Geometry check sheet. Reference: the model listing, model coordinates, mm. A direction names the side the tool comes from. Round coordinates to 2 decimals unless told otherwise and drop trailing zeros. Write each loop counter-clockwise with the first axis right and the second up, starting at its lowest first coordinate (ties: lowest second). Pieces come first, ordered by that corner, then holes. Notation, with made-up numbers: M -17,61 L 38,61 A30 cw 38,92 Z; hole C -8,-28 d11. An arc over 180 degrees is marked long. One line per item, written item: value. Start each with the question number.
1. Section check A-A (y = -69.5). Record the boundary of the cut face in (x, z).
2. Scan lines: probe 1 along X at (y, z) = (-54.5, 4.5); probe 2 along Y at (x, z) = (100, 5.5); probe 3 along Y at (x, z) = (101.6, 7.75). Record each from-to range of solid material in increasing order. Write a range as [from, to].
3. Access from +Z, -Z, +X, -X, +Y, -Y to the whole of each face (thin tool, end or side, straight path). Record for faces 4 (the flat face through (230, 107.95, 6)), 5 (the flat face through (2, 215.9, 6)), 6 (the flat face through (-227, 107.95, 6)), 7 (the flat face through (-95.43, -12.88, 6.26)).
4. Section check B-B (x = 195). Record the boundary of the cut face in (y, z), and give its area (3 significant figures).
5. Depth check by flat-ended pin: P1, Ø6, axis at x = -239.61, y = 101.6, coming from the -Z side; P2, Ø6, axis at x = 317.5, y = 33.87, coming from the +Z side; P3, Ø4, axis at x = -114.3, y = -53.77, coming from the +Z side; P4, Ø4, axis at x = 191, z = 7.5, coming from the +Y side. Enter the tip coordinate at first touch or a pass-through.
6. Section check C-C (z = 8.75). Count the separate pieces of the cut face and the enclosed holes in it, and give its area (3 significant figures).
7. Release check for a two-part mould opening along X. For faces 1 (the flat face through (-323.85, 2, 6)), 2 (the flat face through (107.95, -66, 6)), 3 (the flat face through (214, -107.95, 6)) record: pulls with the +X half, pulls with the -X half, needs draft (parallel to the pull), parting line crosses it, or undercut.
from build123d import *

# Parameters (mm, degrees)
F0_R           = 27.94
F1_DEPTH       = 12.7
F3_D           = 4.7625
F3_CSINK_D     = 7.9375
F3_CSINK_ANGLE = 85
F4_SIZE        = 1.5875


with BuildPart() as f1:
    # F0 (on Top) → F1 (new body)
    with BuildSketch(Plane.XY):
        Polygon((-82.55, 0), (82.55, 0), (107.95, -25.4), (107.95, -107.95), (323.85, -107.95), (323.85, 107.95), (133.35, 107.95), (107.95, 133.35), (107.95, 215.9), (-107.95, 215.9), (-107.95, 133.35), (-133.35, 107.95), (-323.85, 107.95), (-323.85, -107.95), (-107.95, -107.95), (-107.95, -25.4), align=None)
        with Locations((0, 107.95)):
            Circle(F0_R, mode=Mode.SUBTRACT)
    extrude(amount=F1_DEPTH)

    # F3 (through all)
    with Locations(Plane.XY.offset(12.7)):
        with Locations((-239.609983, 101.6), (-161.719967, 101.6), (-116.159872, 116.159872), (-101.6, 161.719967), (-101.6, 209.55), (-33.866667, 209.55), (33.866667, 209.55), (101.6, 209.55), (101.6, 161.719967), (116.159872, 116.159872), (161.719967, 101.6), (239.609983, 101.6), (317.5, 33.866667), (317.5, 101.6), (317.5, -33.866667), (317.5, -101.6), (249.766667, -101.6), (182.033333, -101.6), (114.3, -53.769967), (114.3, -101.6), (99.740128, -8.209872), (54.180033, 6.35), (0, 6.35), (-54.180033, 6.35), (-99.740128, -8.209872), (-114.3, -53.769967), (-114.3, -101.6), (-182.033333, -101.6), (-249.766667, -101.6), (-317.5, -101.6), (-317.5, -33.866667), (-317.5, 33.866667), (-317.5, 101.6)):
            CounterSinkHole(F3_D / 2, F3_CSINK_D / 2, counter_sink_angle=F3_CSINK_ANGLE)

    # F4
    f4_edges = [f1.edges().sort_by_distance(p)[0] for p in [
        (-27.94, 107.95, 12.7),
    ]]
    chamfer(f4_edges, length=F4_SIZE)


solid = f1.part
Result sheet:
1. outline: M -323.85,0 L -107.95,0 L -107.95,12.7 L -323.85,12.7 Z; M 107.95,0 L 323.85,0 L 323.85,12.7 L 107.95,12.7 Z
2. probe 1: x = [-323.85, -116.57], [-112.03, -107.95], [107.95, 112.03], [116.57, 323.85]
2. probe 2: y = [-17.45, -10.58], [-5.84, 159.96], [163.48, 207.79], [211.31, 215.9]
2. probe 3: y = [-19.05, -9.7], [-6.72, 159.34], [164.1, 207.17], [211.93, 215.9]
3. face 4: +Z, -Z, +X, +Y
3. face 5: +Z, -Z, +X, -X, +Y
3. face 6: +Z, -Z, -X, +Y
3. face 7: +Z, -Z, -Y
4. outline: M -107.95,0 L 107.95,0 L 107.95,12.7 L -107.95,12.7 Z
4. area: 2,740 mm2
5. P1: stops at z = 0
5. P2: stops at z = 11.65
5. P3: passes through
5. P4: stops at y = 107.95
6. separate pieces: 1
6. enclosed holes: 34
6. area: 138,000 mm2
7. face 1: pulls with the -X half
7. face 2: undercut
7. face 3: needs draft
